from build123d import *

# Parameters (mm, degrees)
SKETCH_1_W          = 10
SKETCH_1_H          = 20
SKETCH_1_W_2        = 7.6
SKETCH_1_H_2        = 17.6
EXTRUDE_1_DEPTH     = 645
SKETCH_2_R          = 2
CUT_EXTRUDE_1_DEPTH = 646.155020131
SKETCH_3_R          = 2
CUT_EXTRUDE_2_DEPTH = 646.329373266


with BuildPart() as part:
    # ｽｹｯﾁ1 → 押し出し-薄板1 (new body)
    with BuildSketch(Plane(origin=(0, 0, 0), x_dir=(0, 0, -1), z_dir=(1, 0, 0))):
        Rectangle(SKETCH_1_W, SKETCH_1_H)
        Rectangle(SKETCH_1_W_2, SKETCH_1_H_2, mode=Mode.SUBTRACT)
    extrude(amount=EXTRUDE_1_DEPTH)

    # ｽｹｯﾁ2 → ｶｯﾄ - 押し出し1 (cut, through all)
    with BuildSketch(Plane.XY.offset(5)):
        with Locations((163.5, -5)):
            Circle(SKETCH_2_R)
        with Locations(Location((163.5, 5, 0), (0, 0, 90))):
            Circle(SKETCH_2_R)
        with Locations((637.5, 5)):
            Circle(SKETCH_2_R)
        with Locations(Location((637.5, -5, 0), (0, 0, 90))):
            Circle(SKETCH_2_R)
        with Locations((7.5, -5)):
            Circle(SKETCH_2_R)
        with Locations(Location((7.5, 5, 0), (0, 0, 90))):
            Circle(SKETCH_2_R)
    extrude(amount=-CUT_EXTRUDE_1_DEPTH, mode=Mode.SUBTRACT)

    # ｽｹｯﾁ3 → ｶｯﾄ - 押し出し2 (cut, through all)
    with BuildSketch(Plane(origin=(0, 10, 0), x_dir=(1, 0, 0), z_dir=(0, 1, 0))):
        with Locations(Location((20, 0, 0), (0, 0, 270))):
            Circle(SKETCH_3_R)
        with Locations(Location((625, 0, 0), (0, 0, 270))):
            Circle(SKETCH_3_R)
        with Locations(Location((310, 0, 0), (0, 0, 270))):
            Circle(SKETCH_3_R)
        with Locations(Location((335, 0, 0), (0, 0, 270))):
            Circle(SKETCH_3_R)
    extrude(amount=-CUT_EXTRUDE_2_DEPTH, mode=Mode.SUBTRACT)


solid = part.part
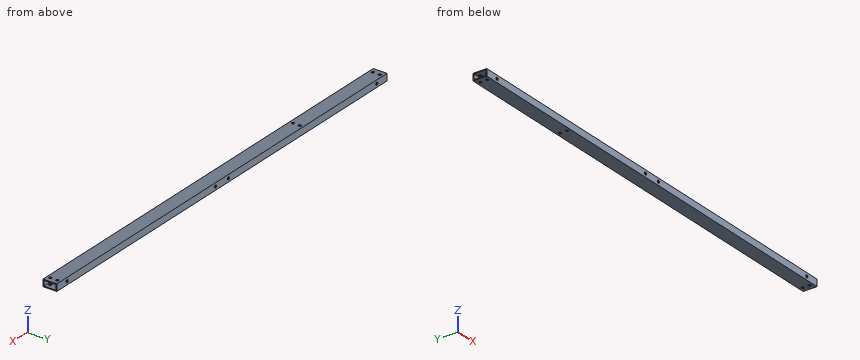
Design review of the part built by this model. Coordinates are the model's own, in mm. Round coordinates to 2 decimals unless told otherwise and drop trailing zeros. Loops run counter-clockwise (first coordinate to the right, second up) from the corner with the lowest first, then second, coordinate; pieces in that order, holes last. Notation, with made-up numbers: M -8.5,33 L 23.5,33 A15 ccw 23.5,50 Z; hole C 11.5,53.25 d11. An arc over 180 degrees is marked long. Answer as a JSON object with one key per item and string values.
Item 1: We need section A-A on x = 442. Give the boundary of the cut face in (y, z).
Answer sheet:
{"outline": "M -10,-5 L 10,-5 L 10,5 L -10,5 Z; hole M -8.8,-3.8 L 8.8,-3.8 L 8.8,3.8 L -8.8,3.8 Z"}
Item 2: Clearance check with a flat-ended pin moving along its axis: P1, Ø3.5, axis at x = 20, z = 0, coming from the +Y side. State where the tip first meets the part, or that it passes through.
Answer sheet:
{"P1": "passes through"}
Item 3: Wall thickness on L1, parallel to X at y = 9.75, z = 0; L2, parallel to Y at x = 637.5, z = 4.75; L3, parallel to Z at x = 550, y = 2.5: over which ranges is each line inside the solid? List them lowest first. Write a range as from..to.
Answer sheet:
{"L1": "x = 0..18, 22..308, 312..333, 337..623, 627..645", "L2": "y = -10..-7, -3..3, 7..10", "L3": "z = -5..-3.8, 3.8..5"}
Item 4: We need section B-B on z = 0. State how many separate pieces and enclosed holes the cut face has, and give its area (3 significant figures).
Answer sheet:
{"separate pieces": "10", "enclosed holes": "0", "area": "1,510 mm^2"}
